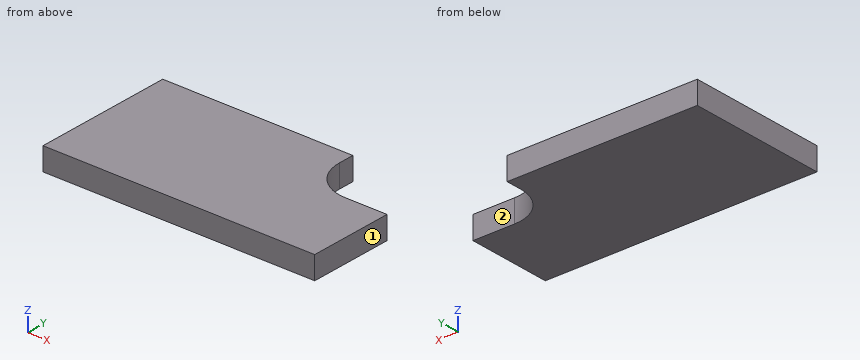
from build123d import *

# Parameters (mm, degrees)
BOSS_EXTRUDE1_DEPTH = 5.5
BOSS_EXTRUDE2_DEPTH = 7
SKETCH3_W           = 105
SKETCH3_H           = 14.2
CUT_EXTRUDE1_DEPTH  = 177.40932515


with BuildPart() as part:
    # Sketch1 → Boss-Extrude1 (new body)
    with BuildSketch(Plane.XY):
        with BuildLine():
            Line((127, 47), (150, 47))
            Line((150, 47), (150, 0))
            Line((150, 0), (0, 0))
            Line((0, 0), (0, 69))
            Line((0, 69), (0, 92))
            Line((0, 92), (105, 92))
            Line((105, 92), (105, 69))
            ThreePointArc((105, 69), (111.443650814, 53.443650814), (127, 47))
        make_face()
    extrude(amount=BOSS_EXTRUDE1_DEPTH)

    # Sketch2 → Boss-Extrude2 (add)
    with BuildSketch(Plane.XY.offset(5.5)):
        with BuildLine():
            Line((0, 92), (0, 0))
            Line((0, 0), (150, 0))
            Line((150, 0), (150, 47))
            Line((150, 47), (127, 47))
            ThreePointArc((127, 47), (111.443650814, 53.443650814), (105, 69))
            Line((105, 69), (105, 92))
            Line((105, 92), (0, 92))
        make_face()
    extrude(amount=BOSS_EXTRUDE2_DEPTH)

    # Sketch3 → Cut-Extrude1 (cut, through all)
    with BuildSketch(Plane.XY.offset(12.5)):
        with Locations((52.5, 84.9)):
            Rectangle(SKETCH3_W, SKETCH3_H)
    extrude(amount=-CUT_EXTRUDE1_DEPTH, mode=Mode.SUBTRACT)


solid = part.part
Can you work these out from the model? Positions are in its coordinate system, mm. Face numbers are marked on the shaded views. A direction names the side the tool comes from. Give positions to 0.01 mm unless a question says otherwise; leave off trailing zeros. Write each loop counter-clockwise with the first axis right and the second up, starting at its lowest first coordinate (ties: lowest second). Pieces come first, ordered by that corner, then holes. Notation, with made-up numbers: (25, 61.25) -> (30, 61.25) arc R14 cw to (30, 81.25) -> close; hole circle Ø3 at (11.5, 73). An arc over 180 degrees is marked (long way). Answer as a JSON object with one key per item and string values. Group by question number.
Item 1: For the marked faces 1 and 2, which set-ups out of +Z, -Z, +X, -X, +Y, -Y let a thin tool reach every point of the face, with its end or its side?
Item 2: Suppose I cut it at A-A (z = 7.25). Please give me the cut outline in (x, y), plus the area to 3 significant figures.
Item 3: Suppose I cut it at B-B (y = 63). Please give me the cut outline in (x, z), plus the area to 3 significant figures.
Item 4: Please list where these lines run through material, in increasing order: line 1 (X direction, y = 73.5, z = 5.5); line 2 (Y direction, x = 140.5, z = 8.25); line 3 (X direction, y = 58, z = 6.25). Write a range as [from, to].
Item 5: Suppose I cut it at C-C (y = 55). Please give me the cut outline in (x, z).
Item 6: I'm going to push flat-ended pins straight in: P1, Ø6, axis at y = 16, z = 6, coming from the -X side; P2, Ø7, axis at y = 74.5, z = 3.5, coming from the +X side; P3, Ø6, axis at x = 139.5, z = 8.5, coming from the +Y side. Where does each tip first touch, or does it pass through?
Findings:
{
 "1": {"face 1": "+Z, -Z, +X, +Y, -Y", "face 2": "+Z, -Z, +X, +Y"},
 "2": {"outline": "(0, 0) -> (150, 0) -> (150, 47) -> (127, 47) arc R22 cw to (105, 69) -> (105, 77.8) -> (0, 77.8) -> close", "area": "10,400 mm²"},
 "3": {"outline": "(0, 0) -> (105.83, 0) -> (105.83, 12.5) -> (0, 12.5) -> close", "area": "1,320 mm²"},
 "4": {"line 1": "x = [0, 105]", "line 2": "y = [0, 47]", "line 3": "x = [0, 107.95]"},
 "5": {"outline": "(0, 0) -> (110.03, 0) -> (110.03, 12.5) -> (0, 12.5) -> close"},
 "6": {"P1": "stops at x = 0", "P2": "stops at x = 105", "P3": "stops at y = 47"}
}
